Design review of the part built by this model. Coordinates are the model's own, in mm. A direction names the side the tool comes from. Round coordinates to 2 decimals unless told otherwise and drop trailing zeros. Loops run counter-clockwise (first coordinate to the right, second up) from the corner with the lowest first, then second, coordinate; pieces in that order, holes last. Notation, with made-up numbers: M 43,24 L 70,24 A17 ccw 70,43 Z; hole C 81.25,11 d11. An arc over 180 degrees is marked long. One line per item, written item: value. Start each with the question number.
Item 1: We need section C-C (z = 12.5). Write out the cut boundary in (x, y).
Item 2: We need section D-D (z = -5.5). Write out the cut boundary in (x, y).
Item 3: For line 1 along Y through (x, z) = (0, 6.75); line 2 along Y through (x, z) = (0, -2); line 3 along Z through (x, y) = (-3, 4), list the stretches that pass through material, from the lowest coordinate up.
Item 4: For faces 1 (the flat face through (-3.4, 12.3, 15)), 2 (the cylindrical face through (-14.985, 0.66, 9.93)), list the 3-axis set-ups (+Z, -Z, +X, -X, +Y, -Y) from which the entire face can be reached by the end or side of a thin tool; tool diameter is ignored.
Item 5: Clearance check with flat-ended pins moving along their axes: pin 1 (1 mm diameter, centred on y = 11, z = 8.5, fed in from +X); pin 2 (2 mm diameter, centred on y = -12, z = 4.5, fed in from -X); pin 3 (6 mm diameter, centred on y = -10, z = 7.5, fed in from +X). State where each tip first meets the part, or that it passes through.
Item 6: Mouldability with a two-part tool opening along Y and no side actions: class faces 3 (the flat face through (0, 0, -10)), 4 (the cylindrical face through (-4.336, -19.524, -5.07)), 5 (the flat face through (0, 0, 0)) as released by +Y, released by -Y, zero draft, split by the parting line, or undercut.
from build123d import *

# Parameters (mm, degrees)
SKETCH1_R           = 15
SKETCH1_R_2         = 12.5
BOSS_EXTRUDE1_DEPTH = 15
BOSS_EXTRUDE2_START = -10
SKETCH1_3_R         = 20
SKETCH1_3_R_2       = 15
SKETCH1_3_R_3       = 12.5
BOSS_EXTRUDE2_DEPTH = 10
CHAMFER1_SIZE       = 5


with BuildPart() as part:
    # Sketch1 → Boss-Extrude1 (new body)
    with BuildSketch(Plane.XY):
        Circle(SKETCH1_R)
        Circle(SKETCH1_R_2, mode=Mode.SUBTRACT)
    extrude(amount=BOSS_EXTRUDE1_DEPTH)

    # Sketch1<3> → Boss-Extrude2 (add)
    # profile 1 of 3: a face of its own
    with BuildSketch(Plane.XY.offset(BOSS_EXTRUDE2_START)):
        Circle(SKETCH1_3_R)
        Circle(SKETCH1_3_R_2, mode=Mode.SUBTRACT)
    # profile 2 of 3: a face of its own
    with BuildSketch(Plane.XY.offset(BOSS_EXTRUDE2_START)):
        Circle(SKETCH1_3_R_2)
        Circle(SKETCH1_3_R_3, mode=Mode.SUBTRACT)
    # profile 3 of 3: a face of its own
    with BuildSketch(Plane.XY.offset(BOSS_EXTRUDE2_START)):
        Circle(SKETCH1_3_R_3)
    extrude(amount=BOSS_EXTRUDE2_DEPTH)

    # Chamfer1
    chamfer1_edges = [part.edges().sort_by_distance(p)[0] for p in [
        (-15, 0, 0),
    ]]
    chamfer(chamfer1_edges, length=CHAMFER1_SIZE - 0.0001)  # a hair under: the kernel refuses the full size


solid = part.part
A:
1. outline: C 0,0 d30; hole C 0,0 d25
2. outline: C 0,0 d40
3. line 1: -15 to -12.5, 12.5 to 15
3. line 2: -20 to 20
3. line 3: -10 to 0
4. face 1: +Z, +X, -X, +Y, -Y
4. face 2: +Z
5. pin 1: x = 10.71
5. pin 2: x = -11.65
5. pin 3: x = 13.27
6. face 3: zero draft
6. face 4: split by the parting line
6. face 5: undercut
